from build123d import *

# Parameters (mm, degrees)
ESQUISSE1_W             = 140
ESQUISSE1_H             = 80
EXTRUSION1_DEPTH        = 6
CONG_1_R                = 10
ESQUISSE2_R             = 3.25
ENL_V_MAT_EXTRU_1_DEPTH = 90.643739324
ESQUISSE5_R             = 1.05
ENL_V_MAT_EXTRU_2_DEPTH = 1
EXTRUSION2_DEPTH        = 6
ESQUISSE7_R             = 1.05
ENL_V_MAT_EXTRU_3_DEPTH = 95.223768892


with BuildPart() as part:
    # Esquisse1 → Extrusion1 (new body)
    with BuildSketch(Plane.XY):
        with Locations((10, 0)):
            Rectangle(ESQUISSE1_W, ESQUISSE1_H)
    extrude(amount=EXTRUSION1_DEPTH)

    # Congé1
    cong_1_edges = [part.edges().sort_by_distance(p)[0] for p in [
        (-60, 40, 3),
        (80, 40, 3),
    ]]
    fillet(cong_1_edges, radius=CONG_1_R)

    # Esquisse2 → Enlèv. mat.-Extru.1 (cut, through all)
    with BuildSketch(Plane.XY.offset(6)):
        with Locations((10, 10)):
            Circle(ESQUISSE2_R)
    extrude(amount=-ENL_V_MAT_EXTRU_1_DEPTH, mode=Mode.SUBTRACT)

    # Esquisse5 → Enlèv. mat.-Extru.2 (cut)
    with BuildSketch(Plane(origin=(0, 0, 0), x_dir=(-1, 0, 0), z_dir=(0, 0, -1))):
        with Locations((19.77, 14.8)):
            Circle(ESQUISSE5_R)
        with Locations((19.77, 5.3)):
            Circle(ESQUISSE5_R)
    extrude(amount=-ENL_V_MAT_EXTRU_2_DEPTH, mode=Mode.SUBTRACT)

    # Esquisse6 → Extrusion2 (add)
    with BuildSketch(Plane(origin=(0, 0, 0), x_dir=(-1, 0, 0), z_dir=(0, 0, -1))):
        with BuildLine():
            Line((-50, 40), (30, 40))
            ThreePointArc((30, 40), (-10, 49.417796635), (-50, 40))
        make_face()
    extrude(amount=-EXTRUSION2_DEPTH)

    # Esquisse7 → Enlèv. mat.-Extru.3 (cut, through all)
    with BuildSketch(Plane(origin=(0, 0, 0), x_dir=(-1, 0, 0), z_dir=(0, 0, -1))):
        with Locations((46.75, 10)):
            Circle(ESQUISSE7_R)
    extrude(amount=-ENL_V_MAT_EXTRU_3_DEPTH, mode=Mode.SUBTRACT)


solid = part.part
Design review of the part built by this model. Coordinates are the model's own, in mm. A direction names the side the tool comes from. Round coordinates to 2 decimals unless told otherwise and drop trailing zeros. Loops run counter-clockwise (first coordinate to the right, second up) from the corner with the lowest first, then second, coordinate; pieces in that order, holes last. Notation, with made-up numbers: (27.5, 53) - (84.5, 53) arc R29 cw to (84.5, 89) - close; hole circle Ø11 at (71, -3). An arc over 180 degrees is marked (long way). One line per item, written item: value. Start each with the question number.
1) Consider section D-D on y = 42.5. Give the boundary of the cut face in (x, z), then the cut area to 3 significant figures.
2) Draft analysis for pull direction Y (two halves, no side actions). For faces 3 (the flat face through (9, -40, 3)), 4 (the flat face through (60, 40, 3)), 5 (the cylindrical face through (6.753, 10.143, 3.042)), state which applies: +Y half, -Y half, draft (parallel to the pull), parting line (faces both ways), or undercut.
3) Consider section B-B on z = 2.7. Give the boundary of the cut face in (x, y).
4) To check wall thickness, follow L1, parallel to Y at x = -46.75, z = 3.25; L2, parallel to Y at x = -36, z = 3.85; L3, parallel to X at y = 7, z = 4.8. State the ranges of each line that lie inside material, in increasing order. Write a range as from..to.
5) Consider section C-C on x = -35. Give the boundary of the cut face in (y, z).
6) For faces 1 (the flat face through (-40, 40, 3)), 2 (the flat face through (-60, -5, 3)), list the 3-axis set-ups (+Z, -Z, +X, -X, +Y, -Y) from which the entire face can be reached by the end or side of a thin tool; tool diameter is ignored.
7) Insertion check: pin 1 Ø6 at (x, y) = (10, 10) entering from +Z; pin 2 Ø1.7 at (x, y) = (-19.5, 14.5) entering from -Z; pin 3 Ø3 at (x, z) = (30, 4) entering from +Y; pin 4 Ø3 at (x, z) = (-43, 4) entering from +Y. Each pin has a flat end and moves straight along its axis. Give the tip position at first contact, or say it passes through.
8) Consider section A-A on x = 10. Give the boundary of the cut face in (y, z), then the cut area to 3 significant figures.
Reported:
1. outline: (-24.53, 0) - (44.53, 0) - (44.53, 6) - (-24.53, 6) - close
1. area: 414 mm^2
2. face 3: -Y half
2. face 4: +Y half
2. face 5: undercut
3. outline: (-60, -40) - (80, -40) - (80, 30) arc R10 ccw to (70, 40) - (50, 40) arc R89.65 ccw to (-30, 40) - (-50, 40) arc R10 ccw to (-60, 30) - close; hole circle Ø2.1 at (-46.75, 10); hole circle Ø6.5 at (10, 10)
4. L1: y = -40..8.95, 11.05..40
4. L2: y = -40..40
4. L3: x = -60..8.75, 11.25..80
5. outline: (-40, 0) - (40, 0) - (40, 6) - (-40, 6) - close
6. face 1: +Z, -Z, -X, +Y
6. face 2: +Z, -Z, -X, +Y, -Y
7. pin 1: passes through
7. pin 2: stops at z = 0
7. pin 3: stops at y = 47.49
7. pin 4: stops at y = 40
8. outline: (-40, 0) - (6.75, 0) - (6.75, 6) - (-40, 6) - close; (13.25, 0) - (49.42, 0) - (49.42, 6) - (13.25, 6) - close
8. area: 498 mm^2
